Design review of the part built by this model. Coordinates are the model's own, in mm. A direction names the side the tool comes from. Round coordinates to 2 decimals unless told otherwise and drop trailing zeros. Loops run counter-clockwise (first coordinate to the right, second up) from the corner with the lowest first, then second, coordinate; pieces in that order, holes last. Notation, with made-up numbers: (49.5, 3.5) - (97.5, 3.5) arc R10 cw to (97.5, 14.5) - close; hole circle Ø7 at (-3, 67). An arc over 180 degrees is marked (long way). Return JSON: item names as keys, results as strings. Group by question number.
Autodesk Inventor part; units mm, degrees
ref_plane "YZ Plane" through (0, 0, 0) normal (1, 0, 0) x (0, 1, 0)
ref_plane "XZ Plane" through (0, 0, 0) normal (0, 1, 0) x (-1, 0, 0)
ref_plane "XY Plane" through (0, 0, 0) normal (0, 0, 1) x (1, 0, 0)
sketch "Sketch1" plane through (0, 0, 0) normal (0, 1, 0) x (-1, 0, 0)
  line L0 (-40, -40) -> (40, -40)
  line L1 (40, -40) -> (40, 40)
  line L2 (40, 40) -> (-40, 40)
  line L3 (-40, 40) -> (-40, -40)
  line L4 (-40, -40) -> (40, 40) construction
  line L5 (40, -40) -> (-40, 40) construction
  point P0 (0, 0)
  dimension "d0" = 80
  dimension "d1" = 80
extrude "Extrusion1" add sketch "Sketch1" along normal blind 15
sketch "Sketch2" plane through (0, 15, 0) normal (0, 1, 0) x (1, 0, 0)
  point P0 (0, 0)
  point P1 (0, 0)
hole "Hole1" at (0, 15, 0) direction (0, -1, 0) diameter 58 end through all
sketch "Sketch3" plane through (0, 15, 0) normal (0, 1, 0) x (1, 0, 0)
  arc A0 (0, -37.5) -> (0, 37.5) centre (0, 0) ccw
  line L0 (-40, -40) -> (40, -40)
  line L1 (40, -40) -> (40, 40)
  line L2 (0, -40) -> (40, -40)
  line L3 (40, -40) -> (40, 40)
  line L4 (40, 40) -> (0, 40)
  line L5 (0, 40) -> (0, 37.5)
  line L6 (0, -37.5) -> (0, -40)
  dimension "d11" = 75
extrude "Extrusion2" cut sketch "Sketch3" against normal through all
sketch "Sketch4" plane through (0, 15, 0) normal (0, 1, 0) x (1, 0, 0)
  line L0 (41.8017, 5) -> (26.6036, 5)
  line L1 (26.6036, 5) -> (26.6036, -5)
  line L2 (26.6036, -5) -> (41.8017, -5)
  line L3 (41.8017, -5) -> (41.8017, 5)
  line L4 (41.8017, 5) -> (26.6036, -5) construction
  line L5 (26.6036, 5) -> (41.8017, -5) construction
  point P0 (0, 0)
  point P1 (34.2027, 0)
  dimension "d14" = 10
extrude "Extrusion3" cut sketch "Sketch4" against normal through all
sketch "Sketch5" plane through (0, 15, 0) normal (0, 1, 0) x (1, 0, 0)
  line L0 (28.5657, -5) -> (37.1652, -5)
  line L1 (32.8654, -5) -> (47.8654, -5)
  line L2 (47.8654, -5) -> (47.8654, -10)
  line L3 (47.8654, -10) -> (32.8654, -10)
  line L4 (32.8654, -10) -> (32.8654, -5)
  line L5 (25.4496, 0) -> (55.494, 0)
  line L6 (28.5657, 5) -> (37.1652, 5)
  line L7 (32.8654, 5) -> (47.8654, 5)
  line L8 (47.8654, 5) -> (47.8654, 10)
  line L9 (47.8654, 10) -> (32.8654, 10)
  line L10 (32.8654, 10) -> (32.8654, 5)
  point P0 (0, 0)
  dimension "d17" = 15
  dimension "d18" = 5
extrude "Extrusion4" add sketch "Sketch5" against normal blind 15
fillet "Fillet1" radius 3 2 edges at (47.8654, 7.5, 10) (47.8654, 7.5, -10)
sketch "Sketch6" plane through (36.1421, 0, 10) normal (0, 0, 1) x (1, 0, 0)
  line L0 (8.7234, 15) -> (8.7234, 0)
  point P0 (-36.1421, 0)
  point P1 (4.1079, 7.5)
  dimension "d22" = 4.6155
hole "Hole2" at (40.2499, 7.5, 10) direction (0, 0, -1) diameter 3 end through all
sketch "Sketch7" plane through (-40, 0, -40) normal (-1, 0, 0) x (0, 0, 1)
  line L0 (30, 15) -> (2.5, 15)
  line L1 (0, 0) -> (80, 0)
  line L2 (24.5, 15) -> (55.5, 15)
  line L3 (55.5, 15) -> (55.5, 0)
  line L4 (55.5, 0) -> (24.5, 0)
  line L5 (24.5, 0) -> (24.5, 15)
  line L6 (0, 0) -> (0, 15)
  point P0 (40, 0)
  dimension "d30" = 31
  dimension "d31" = 24.5
extrude "Extrusion5" add sketch "Sketch7" along normal blind 4
sketch "Sketch8" plane through (-40, 0, -40) normal (-1, 0, 0) x (0, 0, 1)
  line L0 (0, 15) -> (0, 0)
  line L1 (24.5, 15) -> (24.5, 0)
  line L2 (0, 15) -> (24.5, 15)
  line L3 (24.5, 15) -> (24.5, 7.5)
  line L4 (24.5, 7.5) -> (0, 7.5)
  line L5 (0, 7.5) -> (0, 15)
  point P0 (40, 0)
  dimension "d34" = 7.5
extrude "Extrusion6" add sketch "Sketch8" along normal blind 16
properties part number "Clamp" material "PC/ABS Plastic"
Q1. Add section C-C, the plane y = 3. State the section outline as (x, z) points.
Q2. Insertion check: pin 1 Ø3 at (x, y) = (-42.5, 3) entering from -Z; pin 2 Ø0.8 at (y, z) = (4, 38.5) entering from +X; pin 3 Ø2 at (y, z) = (6, 25) entering from +X. Each pin has a flat end and moves straight along its axis. Give the tip position at first contact, or say it passes through.
Q3. For line 1 (X direction, y = 7.5, z = 6.6); line 2 (X direction, y = 7.5, z = -6.25); line 3 (X direction, y = 7.75, z = 21), list the stretches that pass through material, from the lowest coordinate up.
Q4. Draft analysis for pull direction Y (two halves, no side actions). For faces 5 (the cylindrical face through (22.978, 7.605, -29.635)), 6 (the flat face through (-26, 15, -18)), 7 (the cylindrical face through (38.763, 7.695, -7.535)), state which applies: pulls with the +Y half, pulls with the -Y half, needs draft (parallel to the pull), parting line crosses it, or undercut.
Q5. Add section A-A, the plane z = 20.5. State the section outline as (x, y) points, plus the area to 3 significant figures.
Q6. Tool access review of faces 1 (the flat face through (-40, 4, -28)), 2 (the flat face through (-42, 8, 15.5)), 3 (the flat face through (41, 9, -10)), 4 (the flat face through (41, 9, 10)): name each direction out of +Z, -Z, +X, -X, +Y, -Y from which nothing blocks a thin tool from reaching the whole face with its end or side.
Q7. Add section B-B, the plane x = 15.5. State the section outline as (y, z) points, plus the area to 3 significant figures.
Q8. Add section D-D, the plane x = -42. State the section outline as (y, z) points.
Evaluation:
{
 "1": {"outline": "(-44, -15.5) - (-40, -15.5) - (-40, -40) - (0, -40) - (0, -37.5) arc R37.5 ccw to (36.14, -10) - (44.87, -10) arc R3 ccw to (47.87, -7) - (47.87, -5) - (28.57, -5) arc R29 cw (long way) to (28.57, 5) - (47.87, 5) - (47.87, 7) arc R3 ccw to (44.87, 10) - (36.14, 10) arc R37.5 ccw to (0, 37.5) - (0, 40) - (-40, 40) - (-40, 15.5) - (-44, 15.5) - close"},
 "2": {"pin 1": "z = -15.5", "pin 2": "x = 0", "pin 3": "x = 28.81"},
 "3": {"line 1": "-44 to -28.24, 28.24 to 38.75, 41.75 to 47.87", "line 2": "-44 to -28.32, 28.32 to 38.75, 41.75 to 47.87", "line 3": "-40 to -20, 20 to 31.07"},
 "4": {"face 5": "needs draft", "face 6": "pulls with the +Y half", "face 7": "undercut"},
 "5": {"outline": "(-40, 0) - (-20.51, 0) - (-20.51, 15) - (-40, 15) - close; (20.51, 0) - (31.4, 0) - (31.4, 15) - (20.51, 15) - close", "area": "456 mm²"},
 "6": {"face 1": "-Z, -X, -Y", "face 2": "+Z, -X, +Y, -Y", "face 3": "-Z, +X, +Y, -Y", "face 4": "+Z, +X, +Y, -Y"},
 "7": {"outline": "(0, -34.15) - (15, -34.15) - (15, -24.51) - (0, -24.51) - close; (0, 24.51) - (15, 24.51) - (15, 34.15) - (0, 34.15) - close", "area": "289 mm²"},
 "8": {"outline": "(0, -15.5) - (7.5, -15.5) - (7.5, -40) - (15, -40) - (15, 15.5) - (0, 15.5) - close"}
}
